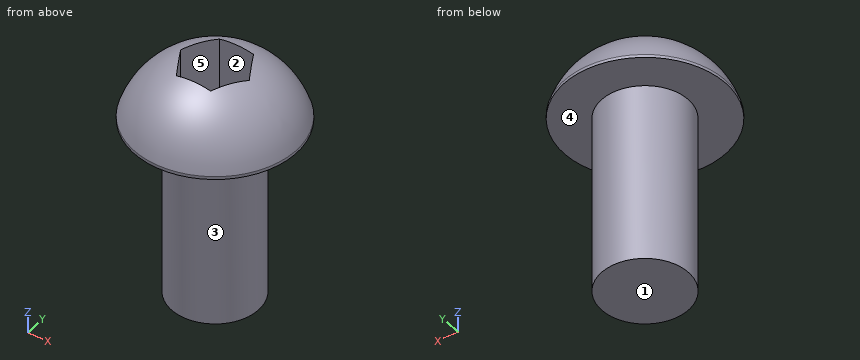
from build123d import *

# Parameters (mm, degrees)
SKETCH1_R           = 1.45
BOSS_EXTRUDE1_DEPTH = 6
SKETCH2_R           = 2.7
BOSS_EXTRUDE2_DEPTH = 0.1
DOME1_FACE_RADIUS   = 2.7
DOME1_HEIGHT        = 2
CUT_EXTRUDE1_DEPTH  = 3.1


with BuildPart() as part:
    # Sketch1 → Boss-Extrude1 (new body)
    with BuildSketch(Plane.XY):
        Circle(SKETCH1_R)
    extrude(amount=BOSS_EXTRUDE1_DEPTH)

    # Sketch2 → Boss-Extrude2 (add)
    with BuildSketch(Plane.XY.offset(6)):
        Circle(SKETCH2_R)
    extrude(amount=BOSS_EXTRUDE2_DEPTH)

    # Dome1: a dome of height H over a round flat face of radius A is a cap of a sphere of radius (A * A + H * H) / (2 * H)
    dome1_r = (DOME1_FACE_RADIUS * DOME1_FACE_RADIUS + DOME1_HEIGHT * DOME1_HEIGHT) / (2 * DOME1_HEIGHT)
    dome1_base = Plane((0, 0, 6.1), z_dir=(0, 0, 1))
    with Locations(dome1_base.offset(DOME1_HEIGHT - dome1_r)):
        dome1_ball = Sphere(dome1_r, mode=Mode.PRIVATE)
    add(split(dome1_ball, bisect_by=dome1_base, keep=Keep.TOP, mode=Mode.PRIVATE))

    # Sketch3 → Cut-Extrude1 (cut, through all)
    with BuildSketch(Plane(origin=(0, 0, 6), x_dir=(-1, 0, 0), z_dir=(0, 0, -1))):
        Polygon((-0.577350269, 1), (-1.154700538, 0), (-0.577350269, -1), (0.577350269, -1), (1.154700538, 0), (0.577350269, 1), align=None)
    extrude(amount=-CUT_EXTRUDE1_DEPTH, mode=Mode.SUBTRACT)


solid = part.part
The listing builds one solid part. Answer for the finished solid, in the listing's coordinates (mm). Face numbers are marked on the shaded views. A direction names the side the tool comes from. Coordinates: 2 decimals unless noted, no trailing zeros. Write each loop counter-clockwise with the first axis right and the second up, starting at its lowest first coordinate (ties: lowest second). Pieces come first, ordered by that corner, then holes. Notation, with made-up numbers: M 43.25,69 L 102.25,69 A22 cw 102.25,105 Z; hole C 25,-27.5 d9. An arc over 180 degrees is marked long. Put each result on its own line as item: value. Start each with the question number.
1. Consider line 1 (X direction, y = 1.05, z = 1); line 2 (Z direction, x = 0.55, y = 0.05); line 3 (Y direction, x = 0.7, z = 7). Determine where each line is inside the solid, lowest interval first. Write a range as from..to.
2. Which of the six approach directions +Z, -Z, +X, -X, +Y, -Y give full straight-line access (tool end or side, diameter ignored) to the marked faces 1 and 2?
3. A cutting plane is placed at B-B on z = 7. Write down the section's boundary in (x, y).
4. For a pull along Y with two mould halves and no side action, classify the marked faces 3, 4 and 5 as pulls with the +Y half, pulls with the -Y half, needs draft (parallel to the pull), parting line crosses it, or undercut.
5. A cutting plane is placed at D-D on z = 2. Write down the section's boundary in (x, y), then the cut area to 3 significant figures.
6. A cutting plane is placed at C-C on y = 0.1. Write down the section's boundary in (x, z), then the cut area to 3 significant figures.
7. Flat-ended cylindrical pins translate along their axes: P1, Ø2, axis at y = 1, z = 2, coming from the +X side; P2, Ø1, axis at x = 1.5, y = -2, coming from the +Z side. Find the tip coordinate at first contact, or state that the pin passes through.
Resolved:
1. line 1: x = -1..1
1. line 2: z = 0..6
1. line 3: y = -2.12..-0.79, 0.79..2.12
2. face 1: -Z, +X, -X, +Y, -Y
2. face 2: +Z
3. outline: C 0,0 d4.47; hole M -1.15,0 L -0.58,-1 L 0.58,-1 L 1.15,0 L 0.58,1 L -0.58,1 Z
4. face 3: parting line crosses it
4. face 4: needs draft
4. face 5: undercut
5. outline: C 0,0 d2.9
5. area: 6.61 mm2
6. outline: M -2.7,6 L -1.45,6 L -1.45,0 L 1.45,0 L 1.45,6 L 2.7,6 L 2.7,6.1 A2.82 ccw 1.1,7.88 L 1.1,6 L -1.1,6 L -1.1,7.88 A2.82 ccw -2.7,6.1 Z
6. area: 21.4 mm2
7. P1: stops at x = 1.45
7. P2: stops at z = 7.27
